Print and shaded views of the part. All mm, measured from the part's lowest x, y and z. Coordinates: 2 decimals unless noted, no trailing zeros. Loops run counter-clockwise (first coordinate to the right, second up) from the corner with the lowest first, then second, coordinate; pieces in that order, holes last.
1) Saw through at A-A, the plane x = 88. Write the cut outline in (y, z).
2) Pin check, flat tips, straight feed: pin 1 Ø5.5 at (x, z) = (88, 22.5) entering from +Y; pin 2 Ø4 at (x, z) = (76.5, 26) entering from -Y. Stop position of each tip, or through.
3) Saw through at C-C, the plane y = 1.1. Write the cut outline in (x, z).
4) Saw through at B-B, the plane z = 7.5. Write the cut outline in (x, y).
5) Wall check: line 1 along X through (y, z) = (2.7, 7.5); line 2 along Z through (x, y) = (88, 1.75); line 3 along Z through (x, y) = (90.5, 2.5). Give the ranges that are in metal, low to high.
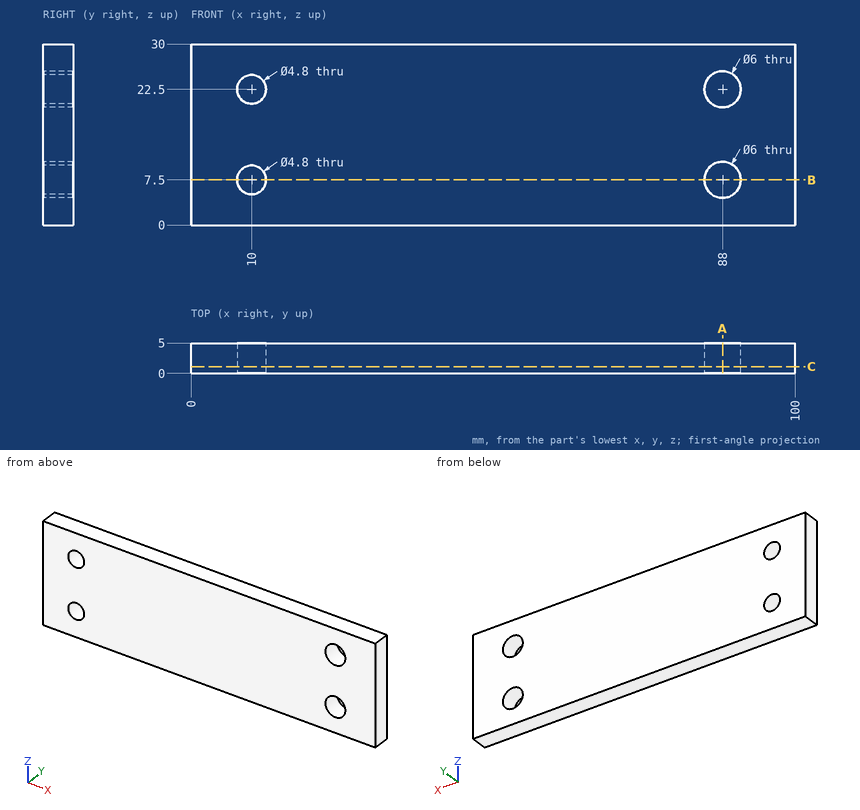
Data:
1. outline: (0, 0) - (5, 0) - (5, 4.5) - (0, 4.5) - close; (0, 10.5) - (5, 10.5) - (5, 19.5) - (0, 19.5) - close; (0, 25.5) - (5, 25.5) - (5, 30) - (0, 30) - close
2. pin 1: passes through
2. pin 2: stops at y = 0
3. outline: (0, 0) - (100, 0) - (100, 30) - (0, 30) - close; hole circle Ø4.8 at (10, 7.5); hole circle Ø4.8 at (10, 22.5); hole circle Ø6 at (88, 7.5); hole circle Ø6 at (88, 22.5)
4. outline: (0, 0) - (7.6, 0) - (7.6, 5) - (0, 5) - close; (12.4, 0) - (85, 0) - (85, 5) - (12.4, 5) - close; (91, 0) - (100, 0) - (100, 5) - (91, 5) - close
5. line 1: x = 0 to 7.6, 12.4 to 85, 91 to 100
5. line 2: z = 0 to 4.5, 10.5 to 19.5, 25.5 to 30
5. line 3: z = 0 to 5.84, 9.16 to 20.84, 24.16 to 30
